```python
from build123d import *

# Parameters (mm, degrees)
F1_DEPTH = 4
F2_SIZE  = 1.5
F3_R     = 1


with BuildPart() as f1:
    # F0 (on Top) → F1 (new body)
    with BuildSketch(Plane.XY):
        Polygon((-2.9, 0), (-2.9, 8.2), (-4.7, 8.2), (-4.7, -1.8), (4.7, -1.8), (4.7, 8.2), (2.9, 8.2), (2.9, 0), align=None)
    extrude(amount=F1_DEPTH)

    # F2
    f2_edges = [f1.edges().sort_by_distance(p)[0] for p in [
        (-2.9, 8.2, 2),
        (2.9, 8.2, 2),
    ]]
    chamfer(f2_edges, length=F2_SIZE)

    # F3
    f3_edges = [f1.edges().sort_by_distance(p)[0] for p in [
        (-2.9, 0, 2),
        (2.9, 0, 2),
        (-4.7, -1.8, 2),
        (4.7, -1.8, 2),
    ]]
    fillet(f3_edges, radius=F3_R)


solid = f1.part
```
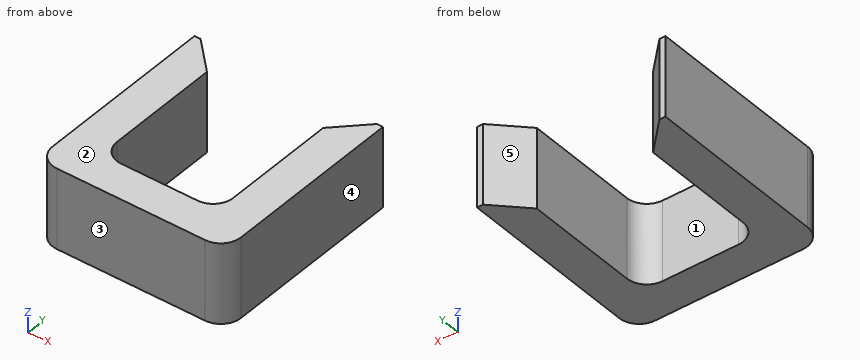
Work out the finished part from the listing and answer in its coordinate system (mm). Face numbers are marked on the shaded views. A direction names the side the tool comes from. Give positions to 0.01 mm unless a question says otherwise; leave off trailing zeros. Loops run counter-clockwise (first coordinate to the right, second up) from the corner with the lowest first, then second, coordinate; pieces in that order, holes last. Notation, with made-up numbers: (86, 89.5) -> (138, 89.5) arc R19 ccw to (138, 93.5) -> close; hole circle Ø10 at (-39, -8). An arc over 180 degrees is marked (long way). Put each result on its own line as item: value. Start each with the question number.
Item 1: The part is cut by section D-D (x = 4). Give the vertices of the cut face in (y, z), then the cut area to 3 significant figures.
Item 2: Which of the six approach directions +Z, -Z, +X, -X, +Y, -Y give full straight-line access (tool end or side, diameter ignored) to the marked faces 1 and 2?
Item 3: The part is cut by section A-A (y = 5). Give the vertices of the cut face in (x, z), then the cut area to 3 significant figures.
Item 4: The mould has two halves that part along X. Classify the marked faces 3, 4 and 5: released by +X, released by -X, zero draft, split by the parting line, or undercut.
Item 5: Find the intervals of material crossed by L1, parallel to X at y = 1.25, z = 0.5; L2, parallel to X at y = 0.25, z = 0.7; L3, parallel to Y at x = -1.75, z = 3, in increasing order. Write a range as [from, to].
Item 6: The part is cut by section C-C (x = -0.75). Give the vertices of the cut face in (y, z), then the cut area to 3 significant figures.
Item 7: The part is cut by section B-B (z = 2.95). Give the vertices of the cut face in (x, y).
Answers below:
1. outline: (-1.75, 0) -> (7.8, 0) -> (7.8, 4) -> (-1.75, 4) -> close
1. area: 38.2 mm2
2. face 1: +Z, -Z, +Y
2. face 2: +Z, +X, -X, +Y, -Y
3. outline: (-4.7, 0) -> (-2.9, 0) -> (-2.9, 4) -> (-4.7, 4) -> close; (2.9, 0) -> (4.7, 0) -> (4.7, 4) -> (2.9, 4) -> close
3. area: 14.4 mm2
4. face 3: zero draft
4. face 4: released by +X
4. face 5: undercut
5. L1: [-4.7, -2.9], [2.9, 4.7]
5. L2: [-4.7, -2.56], [2.56, 4.7]
5. L3: [-1.8, 0]
6. outline: (-1.8, 0) -> (0, 0) -> (0, 4) -> (-1.8, 4) -> close
6. area: 7.20 mm2
7. outline: (-4.7, -0.8) arc R1 ccw to (-3.7, -1.8) -> (3.7, -1.8) arc R1 ccw to (4.7, -0.8) -> (4.7, 8.2) -> (4.4, 8.2) -> (2.9, 6.7) -> (2.9, 1) arc R1 cw to (1.9, 0) -> (-1.9, 0) arc R1 cw to (-2.9, 1) -> (-2.9, 6.7) -> (-4.4, 8.2) -> (-4.7, 8.2) -> close
